```python
from build123d import *

# Parameters (mm, degrees)
RESSALTO_EXTRUS_O1_DEPTH = 3
CORTE_EXTRUS_O3_DEPTH    = 219.215489826
ESBO_O4_W                = 3
ESBO_O4_H                = 30
RESSALTO_EXTRUS_O3_DEPTH = 3


with BuildPart() as part:
    # Esboço1 → Ressalto-extrusão1 (new body)
    with BuildSketch(Plane.XY):
        Polygon((-80, -200), (-55, -200), (-55, -203), (-25, -203), (-25, -200), (25, -200), (25, -203), (55, -203), (55, -200), (80, -200), (80, 200), (-80, 200), align=None)
    extrude(amount=RESSALTO_EXTRUS_O1_DEPTH)

    # Esboço2 → Corte-extrusão3 (cut, through all)
    with BuildSketch(Plane.XY.offset(3)):
        Polygon((0, 200), (0, 170), (3, 170), (3, 140), (0, 140), (0, 107.5), (3, 107.5), (3, 77.5), (0, 77.5), (0, 45), (3, 45), (3, 15), (0, 15), (0, -15), (3, -15), (3, -45), (0, -45), (0, -77.5), (3, -77.5), (3, -107.5), (0, -107.5), (0, -140), (3, -140), (3, -170), (0, -170), (0, -200), (25, -200), (25, -203), (55, -203), (55, -200), (80, -200), (80, 200), align=None)
    extrude(amount=-CORTE_EXTRUS_O3_DEPTH, mode=Mode.SUBTRACT)

    # Esboço4 → Ressalto-extrusão3 (add)
    with BuildSketch(Plane.XY.offset(3)):
        with Locations((-81.5, 155)):
            Rectangle(ESBO_O4_W, ESBO_O4_H)
        with Locations((-81.5, 92.5)):
            Rectangle(ESBO_O4_W, ESBO_O4_H)
        with Locations((-81.5, 30)):
            Rectangle(ESBO_O4_W, ESBO_O4_H)
        with Locations((-81.5, -30)):
            Rectangle(ESBO_O4_W, ESBO_O4_H)
        with Locations((-81.5, -92.5)):
            Rectangle(ESBO_O4_W, ESBO_O4_H)
        with Locations((-81.5, -155)):
            Rectangle(ESBO_O4_W, ESBO_O4_H)
    extrude(amount=-RESSALTO_EXTRUS_O3_DEPTH)


solid = part.part
```
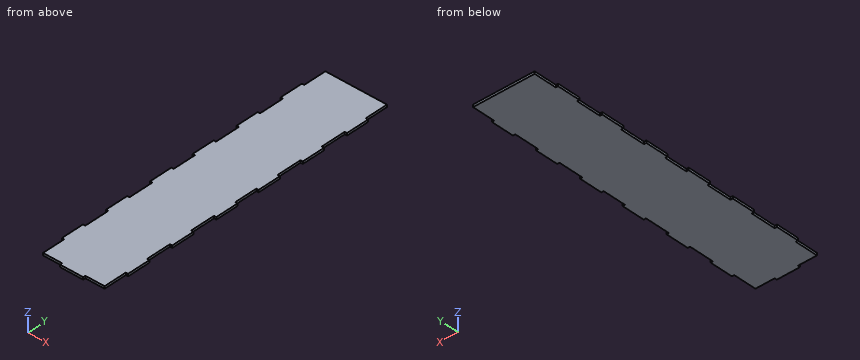
Here's how the part is built. I have some questions about the finished solid (model axes, mm). Give positions to 0.01 mm unless a question says otherwise; leave off trailing zeros. Write each loop counter-clockwise with the first axis right and the second up, starting at its lowest first coordinate (ties: lowest second). Pieces come first, ordered by that corner, then holes. Notation, with made-up numbers: (-13.5, 77.5) -> (33.5, 77.5) arc R11 cw to (33.5, 83.5) -> close; hole circle Ø1 at (-6, 38.5). An arc over 180 degrees is marked (long way). Use one line per item in the form item = value.
1) I'm going to push flat-ended pins straight in: pin 1 (1.5 mm diameter, centred on y = 118.5, z = 1, fed in from +X); pin 2 (0.9 mm diameter, centred on x = 2, z = 1.5, fed in from -Y); pin 3 (1.5 mm diameter, centred on x = 1.5, z = 1, fed in from +Y). Where does each tip first touch, or does it pass through?
Verdict:
pin_1 = 0
pin_2 = -170
pin_3 = 170
2) If I drill on L1, parallel to Y at x = -59, z = 1.35; L2, parallel to X at y = 11, z = 0.6, over which ranges is the centre line in solid material (lowest first)? Write a range as [from, to].
Verdict:
L1 = [-200, 200]
L2 = [-80, 0]
3) Suppose I cut it at A-A (y = 69). Please give me the cut outline in (x, z), and give its area (3 significant figures).
Verdict:
outline = (-80, 0) -> (0, 0) -> (0, 3) -> (-80, 3) -> close
area = 240 mm2
